Here's the drawing with two shaded views (mm, measured from the low corner). I have some questions. A direction names the side the tool comes from. Round coordinates to 2 decimals unless told otherwise and drop trailing zeros. Write each loop counter-clockwise with the first axis right and the second up, starting at its lowest first coordinate (ties: lowest second). Pieces come first, ordered by that corner, then holes. Notation, with made-up numbers: (63.25, 24.5) -> (102.25, 24.5) arc R17 ccw to (102.25, 41.5) -> close; hole circle Ø4 at (-31, -32). An arc over 180 degrees is marked (long way). Use CSV: the item, a comma, the result in double quotes.
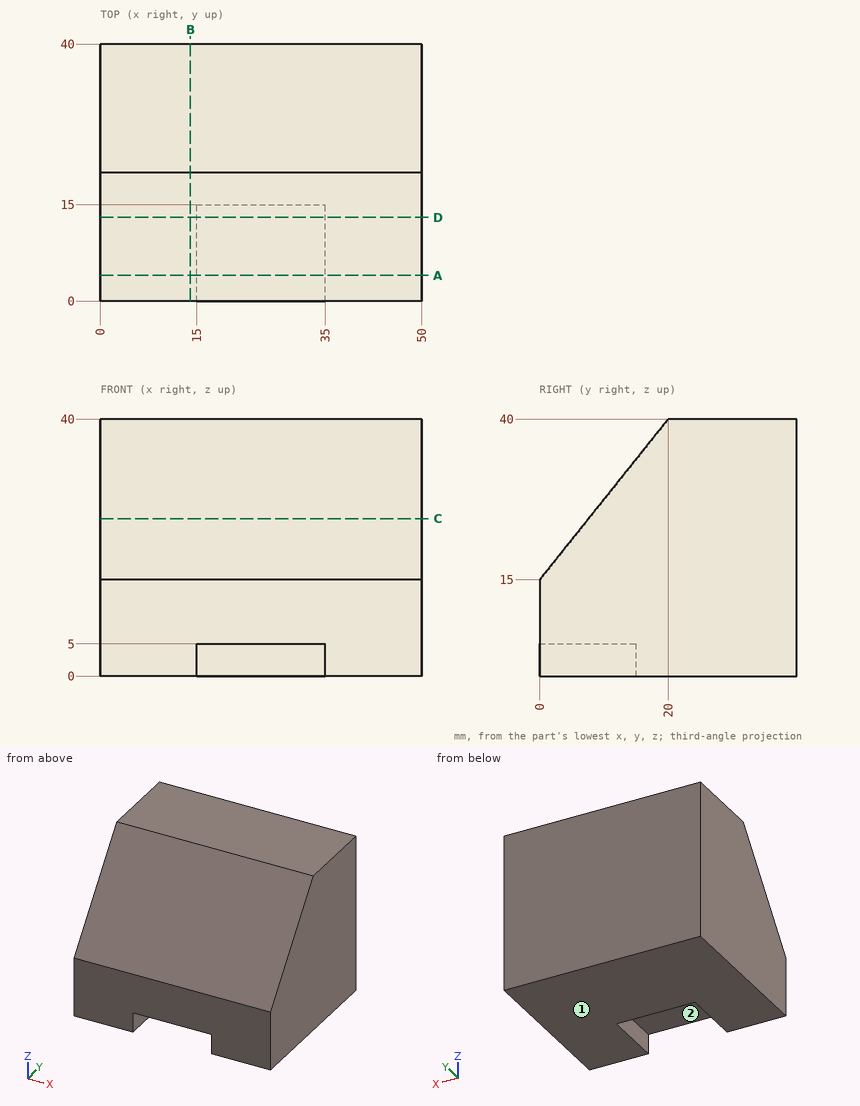
Q1. On a 3-axis mill with a long thin cutter (end or side, diameter ignored), from which of +Z, -Z, +X, -X, +Y, -Y can I reach the whole of each face in a straight line? I mean the marked faces 1 and 2. Say none if no direction works.
Resolved:
face 1,"-Z, +X, -X, +Y, -Y"
face 2,"-Z, -Y"
Q2. Will these pins go through, and if not, where does the flat tip stop? P1, Ø10, axis at y = 10.5, z = 29, coming from the +X side; P2, Ø5, axis at x = 41, z = 21, coming from the -Y side; P3, Ø1.5, axis at x = 23, z = 2, coming from the -Y side; P4, Ø4.5, axis at x = 27, y = 6.5, coming from the -Z side.
Resolved:
P1,"stops at x = 50"
P2,"stops at y = 2.8"
P3,"stops at y = 15"
P4,"stops at z = 5"
Q3. Please list where these lines run through material, in increasing order: probe 1 along Y at (x, z) = (26, 22.5); probe 2 along Z at (x, y) = (30, 4.5) (3 decimals); probe 3 along Y at (x, z) = (16.5, 29).
Resolved:
probe 1,"y = 6 to 40"
probe 2,"z = 5 to 20.625"
probe 3,"y = 11.2 to 40"
Q4. Suppose I cut it at A-A (y = 4). Write out the boundary of the cut face in (x, z), and give its area (3 significant figures).
Resolved:
outline,"(0, 0) -> (15, 0) -> (15, 5) -> (35, 5) -> (35, 0) -> (50, 0) -> (50, 20) -> (0, 20) -> close"
area,"900 mm^2"
Q5. Suppose I cut it at B-B (x = 14). Write out the boundary of the cut face in (y, z), and give its area (3 significant figures).
Resolved:
outline,"(0, 0) -> (40, 0) -> (40, 40) -> (20, 40) -> (0, 15) -> close"
area,"1,350 mm^2"
Q6. Suppose I cut it at D-D (y = 13). Write out the boundary of the cut face in (x, z), and give its area (3 significant figures).
Resolved:
outline,"(0, 0) -> (15, 0) -> (15, 5) -> (35, 5) -> (35, 0) -> (50, 0) -> (50, 31.25) -> (0, 31.25) -> close"
area,"1,460 mm^2"
Q7. Suppose I cut it at C-C (z = 24.5). Write out the boundary of the cut face in (x, y).
Resolved:
outline,"(0, 7.6) -> (50, 7.6) -> (50, 40) -> (0, 40) -> close"
